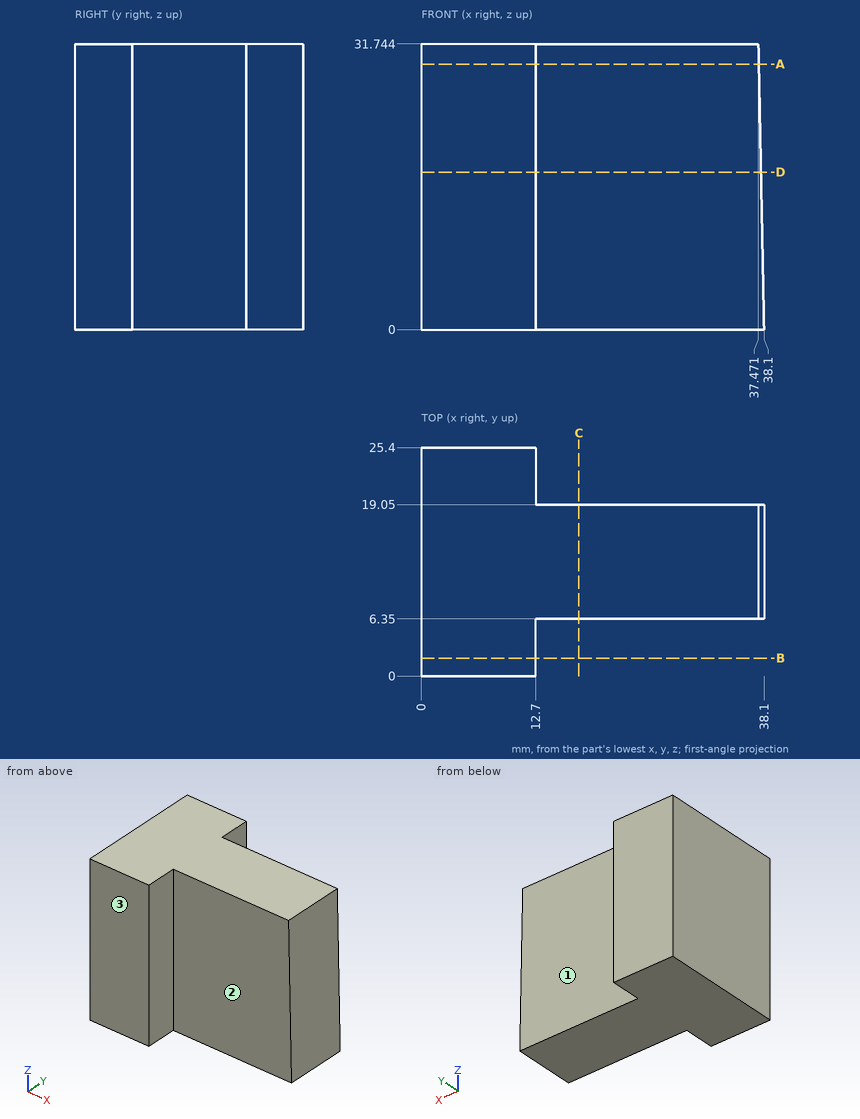
Input: dimensioned drawing with shaded views. Units: mm. Origin: part minimum x, y, z. A direction names the side the tool comes from. Round coordinates to 2 decimals unless told otherwise and drop trailing zeros. Loops run counter-clockwise (first coordinate to the right, second up) from the corner with the lowest first, then second, coordinate; pieces in that order, holes last. Notation, with made-up numbers: M 54.25,-10.5 L 75.25,-10.5 A29 ccw 75.25,9.5 Z; hole C 42,25 d11. An arc over 180 degrees is marked long. Answer in a Markdown table with one row per item. Add a question column.
1. Section D-D (z = 17.5). Output: boundary loops of the cut face in (x, y).
2. Section B-B (y = 2). Output: boundary loops of the cut face in (x, z).
3. Section C-C (x = 17.5). Output: boundary loops of the cut face in (y, z), and give its area (3 significant figures).
4. Contact query for flat-ended pins moving along their axis: pin 1 (10 mm diameter, centred on x = 25, z = 10.5, fed in from +Y); pin 2 (5 mm diameter, centred on y = 21, z = 18.5, fed in from +X) (1 decimal); pin 3 (3 mm diameter, centred on y = 4.5, z = 11, fed in from +X). Output: stop coordinate, or through.
5. Section A-A (z = 29.5). Output: boundary loops of the cut face in (x, y), and give its area (3 significant figures).
6. Ray query, probe 1 along X at (y, z) = (5, 9); probe 2 along Y at (x, z) = (14.5, 30); probe 3 along X at (y, z) = (8.5, 6). Return the intervals inside material, ascending.
7. Set-up query: the marked faces 1, 2 and 3. Return all of +Z, -Z, +X, -X, +Y, -Y with unobstructed straight access to the full face (end or side cutting, diameter ignored); none if empty.
Values follow:
| question | item | result |
|---|---|---|
| 1 | outline | M 0,0 L 12.7,0 L 12.7,6.35 L 37.75,6.35 L 37.75,19.05 L 12.7,19.05 L 12.7,25.4 L 0,25.4 Z |
| 2 | outline | M 0,0 L 12.7,0 L 12.7,31.74 L 0,31.74 Z |
| 3 | outline | M 6.35,0 L 19.05,0 L 19.05,31.74 L 6.35,31.74 Z |
| 3 | area | 403 mm^2 |
| 4 | pin 1 | y = 19.05 |
| 4 | pin 2 | x = 37.8 |
| 4 | pin 3 | x = 12.7 |
| 5 | outline | M 0,0 L 12.7,0 L 12.7,6.35 L 37.52,6.35 L 37.52,19.05 L 12.7,19.05 L 12.7,25.4 L 0,25.4 Z |
| 5 | area | 638 mm^2 |
| 6 | probe 1 | 0 to 12.7 |
| 6 | probe 2 | 6.35 to 19.05 |
| 6 | probe 3 | 0 to 37.98 |
| 7 | face 1 | +Z, -Z, +X, +Y |
| 7 | face 2 | +Z, -Z, +X, -Y |
| 7 | face 3 | +Z, -Z, +X, -X, -Y |
